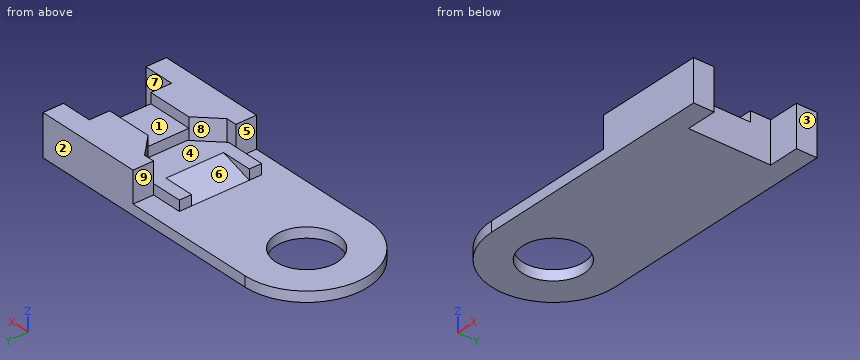
from build123d import *

# Parameters (mm, degrees)
SKETCH2_R               = 30
BOSS_EXTRUDE2_DEPTH     = 10
SKETCH4_W               = 39.74410588
SKETCH4_H               = 80
CUT_EXTRUDE1_DEPTH      = 30
SKETCH5_W               = 105
SKETCH5_H               = 120
BOSS_EXTRUDE3_DEPTH     = 40
SKETCH6_W               = 78.106224714
SKETCH6_H               = 80
CUT_EXTRUDE2_DEPTH      = 30
SKETCH7_W               = 45
SKETCH7_H               = 40
CUT_EXTRUDE3_DEPTH      = 10
CUT_EXTRUDE4_DEPTH      = 30
BOSS_EXTRUDE4_DEPTH     = 10
CUT_EXTRUDE5_DEPTH      = 1
CUT_EXTRUDE5_DEPTH_BACK = 68
SKETCH11_W              = 30
SKETCH11_H              = 10
BOSS_EXTRUDE8_DEPTH     = 12


with BuildPart() as part:
    # Sketch2 → Boss-Extrude2 (new body)
    with BuildSketch(Plane.XY):
        with BuildLine():
            Line((46.207044142, 120), (-84.343419201, 120))
            ThreePointArc((-84.343419201, 120), (-144.343419201, 60), (-84.343419201, 0))
            Line((-84.343419201, 0), (0, 0))
            Line((0, 0), (151.207044142, 0))
            Line((151.207044142, 0), (151.207044142, 120))
            Line((151.207044142, 120), (46.207044142, 120))
        make_face()
        with Locations((-84.343419201, 60)):
            Circle(SKETCH2_R, mode=Mode.SUBTRACT)
    extrude(amount=BOSS_EXTRUDE2_DEPTH)

    # Sketch4 → Cut-Extrude1 (cut)
    with BuildSketch(Plane(origin=(151.207044142, 0, 0), x_dir=(0, 0, -1), z_dir=(1, 0, 0))):
        with Locations((-1.423296347, 60)):
            Rectangle(SKETCH4_W, SKETCH4_H)
    extrude(amount=-CUT_EXTRUDE1_DEPTH, mode=Mode.SUBTRACT)

    # Sketch5 → Boss-Extrude3 (add)
    with BuildSketch(Plane.XY):
        with Locations((98.707044142, 60)):
            Rectangle(SKETCH5_W, SKETCH5_H)
    extrude(amount=BOSS_EXTRUDE3_DEPTH)

    # Sketch6 → Cut-Extrude2 (cut)
    with BuildSketch(Plane(origin=(151.207044142, 0, 0), x_dir=(0, 0, -1), z_dir=(1, 0, 0))):
        with Locations((-16.932746975, 60)):
            Rectangle(SKETCH6_W, SKETCH6_H)
    extrude(amount=-CUT_EXTRUDE2_DEPTH, mode=Mode.SUBTRACT)

    # Sketch7 → Cut-Extrude3 (cut)
    with BuildSketch(Plane.XY.offset(40)):
        with Locations((99.042729198, 60.209092216)):
            Rectangle(SKETCH7_W, SKETCH7_H)
    extrude(amount=-CUT_EXTRUDE3_DEPTH, mode=Mode.SUBTRACT)

    # Sketch8 → Cut-Extrude4 (cut)
    with BuildSketch(Plane.XY.offset(40)):
        Polygon((19.599086243, 100), (56.633635385, 100), (76.633635385, 80), (76.633635385, 40), (56.633635385, 20), (19.599086243, 20), align=None)
    extrude(amount=-CUT_EXTRUDE4_DEPTH, mode=Mode.SUBTRACT)

    # Sketch9 → Boss-Extrude4 (add)
    with BuildSketch(Plane.XY.offset(10)):
        Polygon((46.207044142, 100), (16.207044142, 100), (16.207044142, 20), (46.207044142, 20), (54.69343027, 20), (76.633635385, 41.940205115), (76.633635385, 80), (56.633635385, 100), align=None)
    extrude(amount=BOSS_EXTRUDE4_DEPTH)

    # Sketch10 → Cut-Extrude5 (cut, two sides: drawn at the far end of the back side and taken through both)
    with BuildSketch(Plane.XZ.offset(-20).offset(-CUT_EXTRUDE5_DEPTH_BACK)):
        Polygon((16.207044142, 10), (46.207044142, 20), (16.207044142, 20), align=None)
    extrude(amount=CUT_EXTRUDE5_DEPTH + CUT_EXTRUDE5_DEPTH_BACK, mode=Mode.SUBTRACT)

    # Sketch11 → Boss-Extrude8 (add)
    with BuildSketch(Plane.XZ.offset(-20)):
        with Locations((31.207044142, 15)):
            Rectangle(SKETCH11_W, SKETCH11_H)
    extrude(amount=-BOSS_EXTRUDE8_DEPTH)


solid = part.part
Design review of the part built by this model. Coordinates are the model's own, in mm. Face numbers are marked on the shaded views. A direction names the side the tool comes from. Round coordinates to 2 decimals unless told otherwise and drop trailing zeros. Loops run counter-clockwise (first coordinate to the right, second up) from the corner with the lowest first, then second, coordinate; pieces in that order, holes last. Notation, with made-up numbers: M -36,59 L 17,59 A20 cw 17,70 Z; hole C 83.25,75 d4. An arc over 180 degrees is marked long. Answer as a JSON object with one key per item and string values.
Item 1: Machinability: for the marked faces 5, 6, 7, 8 and 9, which of the approach directions +Z, -Z, +X, -X, +Y, -Y give a long, thin tool a straight path to every point of the face, cutting with its end or side? Answer none if there is none.
Answer sheet:
{"face 5": "+Z, -X, -Y", "face 6": "+Z, -X", "face 7": "+Z, -Z, +X", "face 8": "+Z", "face 9": "+Z, -X, +Y"}
Item 2: We need section A-A on z = 35.5. Give the boundary of the cut face in (x, y).
Answer sheet:
{"outline": "M 46.21,0 L 151.21,0 L 151.21,20 L 121.21,20 L 121.21,40.21 L 76.63,40.21 L 76.63,40 L 56.63,20 L 46.21,20 Z; M 46.21,100 L 56.63,100 L 76.54,80.09 L 76.54,80.21 L 121.21,80.21 L 121.21,100 L 151.21,100 L 151.21,120 L 46.21,120 Z"}
Item 3: The part is to be moulded in two halves that separate along Y. For the marked faces 1, 2, 3 and 4, say which applies: pulls with the +Y half, pulls with the -Y half, needs draft (parallel to the pull), parting line crosses it, or undercut.
Answer sheet:
{"face 1": "undercut", "face 2": "pulls with the +Y half", "face 3": "needs draft", "face 4": "undercut"}
Item 4: Clearance check with flat-ended pins moving along their axes: P1, Ø12, axis at y = 75.5, z = 12.5, coming from the +X side; P2, Ø3, axis at x = 31, z = 13.5, coming from the +Y side; P3, Ø12, axis at x = 103, y = 54, coming from the +Z side; P4, Ø1.5, axis at x = -72, z = 12.5, coming from the +Y side. State where each tip first meets the part, or that it passes through.
Answer sheet:
{"P1": "stops at x = 121.21", "P2": "stops at y = 100", "P3": "stops at z = 30", "P4": "passes through"}
Item 5: Wall thickness on L1, parallel to Y at x = 126.5, z = 17; L2, parallel to Y at x = 23.5, z = 19.5; L3, parallel to Z at x = -107.5, y = 95.5: over which ranges is each line inside the solid? List them lowest first. Write a range as from..to.
Answer sheet:
{"L1": "y = 0..20, 100..120", "L2": "y = 20..32, 88..100", "L3": "z = 0..10"}
Item 6: We need section B-B on y = 60. Give the boundary of the cut face in (x, z).
Answer sheet:
{"outline": "M -144.34,0 L -114.34,0 L -114.34,10 L -144.34,10 Z; M -54.34,0 L 121.21,0 L 121.21,30 L 76.63,30 L 76.63,20 L 46.21,20 L 16.21,10 L -54.34,10 Z"}
Item 7: We need section D-D on x = 36. Give the boundary of the cut face in (y, z).
Answer sheet:
{"outline": "M 0,0 L 120,0 L 120,10 L 100,10 L 100,20 L 88,20 L 88,16.6 L 32,16.6 L 32,20 L 20,20 L 20,10 L 0,10 Z"}
Item 8: We need section C-C on x = -73. Give the boundary of the cut face in (y, z), and give its area (3 significant figures).
Answer sheet:
{"outline": "M 0,0 L 32.23,0 L 32.23,10 L 0,10 Z; M 87.77,0 L 120,0 L 120,10 L 87.77,10 Z", "area": "645 mm^2"}
